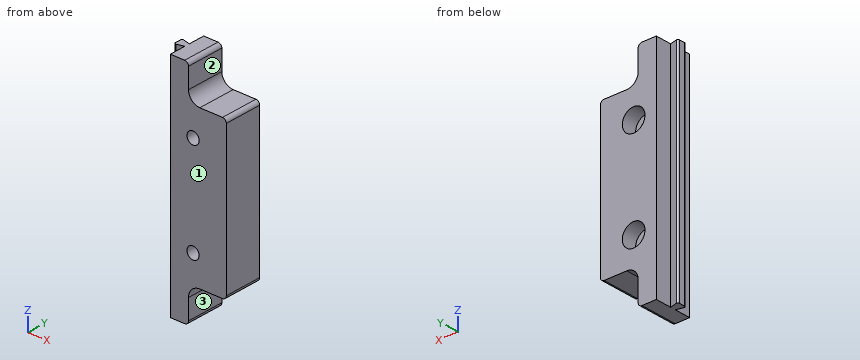
Autodesk Inventor part; units mm, degrees
ref_plane "YZ Plane" through (0, 0, 0) normal (1, 0, 0) x (0, 1, 0)
ref_plane "XZ Plane" through (0, 0, 0) normal (0, 1, 0) x (-1, 0, 0)
ref_plane "XY Plane" through (0, 0, 0) normal (0, 0, 1) x (1, 0, 0)
sketch "Szkic1" plane through (0, 0, 0) normal (0, 1, 0) x (-1, 0, 0)
  line L0 (-1, -9) -> (-6, -9)
  line L1 (-6, -9) -> (-6, -69)
  line L2 (-6, -69) -> (-1, -69)
  line L3 (-1, -69) -> (-1, -9)
  point P0 (0, 0)
  dimension "d0" = 5
  dimension "d1" = 60
extrude "Wyciągnięcie proste1" add sketch "Szkic1" along normal blind 10
sketch "Szkic2" plane through (1, 0, -9) normal (0, 0, 1) x (1, 0, 0)
  line L0 (0, 0) -> (5, 0)
  line L1 (5, 0) -> (5, 10)
  line L2 (0, 10) -> (5, 10)
  line L3 (0, 0) -> (0, 10)
  line L4 (-2.9, 6.95) -> (-2.9, 3.05)
  line L5 (0, 6.2) -> (0, 3.8)
  line L6 (-2.9, 6.95) -> (0, 6.2)
  line L7 (0, 3.8) -> (-2.9, 3.05)
  point P0 (-1, 0)
  point P1 (-2.9, 5)
  point P2 (0, 5)
  point P3 (0, 5)
  point P4 (0, 5)
  dimension "d7" = 3.9
  dimension "d8" = 2.4
  dimension "d9" = 2.9
extrude "Wyciągnięcie proste2" add sketch "Szkic2" against normal up to surface (60 mm away) contours L7 L4 L6 L3
sketch "Szkic3" plane through (0, 10, 0) normal (0, 1, 0) x (1, 0, 0)
  line L0 (16, 18.3) -> (6, 18.3)
  line L1 (6, 18.3) -> (6, 59.7)
  line L2 (6, 59.7) -> (16, 59.7)
  line L3 (16, 59.7) -> (16, 18.3)
  line L4 (6, 9) -> (6, 69)
  point P0 (0, 0)
  point P1 (6, 39)
  point P2 (6, 39)
  point P3 (6, 39)
  dimension "d12" = 41.4
  dimension "d13" = 10
extrude "Wyciągnięcie proste3" add sketch "Szkic3" against normal blind 10
sketch "Szkic4" plane through (0, 10, 0) normal (0, 1, 0) x (1, 0, 0)
  line L0 (6, 9) -> (6, 18.3)
  line L1 (6, 18.3) -> (16, 18.3)
  line L2 (16, 18.3) -> (16, 59.7)
  line L3 (16, 59.7) -> (6, 59.7)
  line L4 (6, 59.7) -> (6, 69)
  line L5 (6, 69) -> (1, 69)
  line L6 (1, 69) -> (1, 9)
  line L7 (1, 9) -> (6, 9)
  line L8 (7, 26) -> (7, 52)
  point P0 (0, 0)
  point P1 (7, 39)
  point P2 (1, 39)
  dimension "d16" = 6
  dimension "d17" = 6
  dimension "d18" = 26
hole "Otwór1" at (7, 10, -26) at (7, 10, -52) direction (0, -1, 0) diameter 3.2 end through all counterbore diameter 6 counterbore depth 4
sketch "Szkic5" plane through (0, 10, 0) normal (0, 1, 0) x (1, 0, 0)
  line L0 (1, 69) -> (-1.9, 69)
  line L1 (6, 69) -> (1, 69)
  line L2 (16, 59.7) -> (6, 59.7)
  line L3 (6, 59.7) -> (6, 69)
  line L4 (16, 18.3) -> (16, 59.7)
  line L5 (6, 18.3) -> (16, 18.3)
  line L6 (1, 9) -> (6, 9)
  line L7 (1, 9) -> (-1.9, 9)
  line L8 (6, 9) -> (6, 18.3)
  line L9 (-1.9, 68.8) -> (1, 68.8)
  line L10 (1, 68.8) -> (5.8, 68.8)
  line L11 (5.8, 68.8) -> (5.8, 59.5)
  line L12 (5.8, 59.5) -> (15.8, 59.5)
  line L13 (15.8, 59.5) -> (15.8, 18.5)
  line L14 (15.8, 18.5) -> (5.8, 18.5)
  line L15 (5.8, 18.5) -> (5.8, 9.2)
  line L16 (5.8, 9.2) -> (1, 9.2)
  line L17 (1, 9.2) -> (-1.9, 9.2)
  line L18 (-1.9, 9) -> (-1.9, 9.2)
  line L19 (-1.9, 68.8) -> (-1.9, 69)
  point P0 (0, 0)
  dimension "d26" = 0.2
extrude "Wyciągnięcie proste4" cut sketch "Szkic5" against normal through all
fillet "Zaokrąglenie1" radius 3 2 edges at (5.8, 5, -18.5) (5.8, 5, -59.5)
fillet "Zaokrąglenie3" radius 1 4 edges at (15.8, 5, -18.5) (15.8, 5, -59.5) (5.8, 5, -9.2) (5.8, 5, -68.8)
sketch "Szkic6" plane through (-1.9, 3.05, -9.2) normal (0, 0, 1) x (1, 0, 0)
  line L0 (6.7, 6.95) -> (6.7, -3.05)
  line L1 (2.9, 6.95) -> (6.7, 6.95)
  line L2 (2.9, 3.15) -> (2.9, 6.95)
  line L3 (0, 3.9) -> (2.9, 3.15)
  line L4 (0, 0) -> (0, 3.9)
  line L5 (2.9, 0.75) -> (0, 0)
  line L6 (2.9, -3.05) -> (2.9, 0.75)
  line L7 (6.7, -3.05) -> (2.9, -3.05)
  line L8 (0.5, 3.2542) -> (3.4, 2.5042)
  line L9 (3.4, 2.5042) -> (3.4, 6.45)
  line L10 (3.4, 6.45) -> (6.2, 6.45)
  line L11 (6.2, 6.45) -> (6.2, -2.55)
  line L12 (6.2, -2.55) -> (3.4, -2.55)
  line L13 (3.4, -2.55) -> (3.4, 1.3958)
  line L14 (3.4, 1.3958) -> (0.5, 0.6458)
  line L15 (0.5, 0.6458) -> (0.5, 3.2542)
  line L16 (2.9, 3.15) -> (2.9, 2.6335)
  line L17 (2.9, 0.75) -> (2.9, -3.05)
  line L18 (2.9, 0.75) -> (2.9, 1.2665)
  point P0 (1.9, -3.05)
  dimension "d32" = 0.5
extrude "Wyciągnięcie proste5" cut sketch "Szkic6" against normal through all contours L16 L8 L15 L14 L18 L5 L4 L3
fillet "Zaokrąglenie4" radius 0.4 2 edges at (-1.4, 3.6958, -39) (-1.4, 6.3042, -39)
properties part number "tyl"
Input: part model. Units: mm. Frame: model coordinates. Face numbers are marked on the shaded views. A direction names the side the tool comes from. Give positions to 0.01 mm unless a question says otherwise; leave off trailing zeros. Loops run counter-clockwise (first coordinate to the right, second up) from the corner with the lowest first, then second, coordinate; pieces in that order, holes last. Notation, with made-up numbers: M 26.5,18 L 62.5,18 A25 cw 62.5,52 Z; hole C 1.25,33.5 d4. An arc over 180 degrees is marked long. Use one line per item in the form item = value.
1. Section query B-B, the plane y = 8. Return the cut outline in (x, z).
Numbers:
outline = M 1,-68.8 L 4.8,-68.8 A1 ccw 5.8,-67.8 L 5.8,-62.5 A3 cw 8.8,-59.5 L 14.8,-59.5 A1 ccw 15.8,-58.5 L 15.8,-19.5 A1 ccw 14.8,-18.5 L 8.8,-18.5 A3 cw 5.8,-15.5 L 5.8,-10.2 A1 ccw 4.8,-9.2 L 1,-9.2 Z; hole C 7,-52 d6; hole C 7,-26 d6
2. Line query: L1, parallel to X at y = 7.4, z = -52; L2, parallel to Z at x = 7, y = 8.9; L3, parallel to Z at x = 9, y = 9. Output: solid intervals per line, ascending.
Numbers:
L1 = 1 to 4, 10 to 15.8
L2 = -60.1 to -55, -49 to -29, -23 to -17.9
L3 = -59.5 to -54.24, -49.76 to -28.24, -23.76 to -18.5
3. Section query A-A, the plane x = 7. Return the cut outline in (y, z), and give its area (3 significant figures).
Numbers:
outline = M 0,-60.1 L 10,-60.1 L 10,-55 L 6,-55 L 6,-53.6 L 0,-53.6 Z; M 0,-50.4 L 6,-50.4 L 6,-49 L 10,-49 L 10,-29 L 6,-29 L 6,-27.6 L 0,-27.6 Z; M 0,-24.4 L 6,-24.4 L 6,-23 L 10,-23 L 10,-17.9 L 0,-17.9 Z
area = 336 mm²
4. Reachability of the marked faces 1, 2 and 3 from +Z, -Z, +X, -X, +Y, -Y: full face, straight path, thin tool, end or side. Return the list, or none.
Numbers:
face_1 = +Z, -Z, +X, -X, -Y
face_2 = +Z, +X, +Y, -Y
face_3 = -Z, +X, +Y, -Y
5. First-contact query: pin 1 (5 mm diameter, centred on x = 11.5, y = 6, fed in from +Z); pin 2 (1.8 mm diameter, centred on x = 8, z = -51.5, fed in from +Y); pin 3 (2.5 mm diameter, centred on x = 7, z = -26, fed in from -Y); pin 4 (6 mm diameter, centred on y = 2.5, z = -65, fed in from +X). Flat tips, straight axial feed; report the tip coordinate or a pass-through.
Numbers:
pin_1 = -18.5
pin_2 = 6
pin_3 = through
pin_4 = 5.84
6. Section query D-D, the plane y = 3. Return the cut outline in (x, z).
Numbers:
outline = M 1,-68.8 L 4.8,-68.8 A1 ccw 5.8,-67.8 L 5.8,-62.5 A3 cw 8.8,-59.5 L 14.8,-59.5 A1 ccw 15.8,-58.5 L 15.8,-19.5 A1 ccw 14.8,-18.5 L 8.8,-18.5 A3 cw 5.8,-15.5 L 5.8,-10.2 A1 ccw 4.8,-9.2 L 1,-9.2 Z; hole C 7,-52 d3.2; hole C 7,-26 d3.2
7. Section query C-C, the plane z = -26. Return the cut outline in (x, y), and give its area (3 significant figures).
Numbers:
outline = M -1.4,4.21 A0.4 ccw -0.9,3.83 L 1,4.32 L 1,0 L 5.4,0 L 5.4,6 L 4,6 L 4,10 L 1,10 L 1,5.68 L -0.9,6.17 A0.4 ccw -1.4,5.79 Z; M 8.6,0 L 15.8,0 L 15.8,10 L 10,10 L 10,6 L 8.6,6 Z
area = 109 mm²
